Model file for the job. Use its own axes, mm. Coordinates: 2 decimals unless noted, no trailing zeros. Order: outer loops, then holes, each group sorted by start corner. A loop starts at its lowest first (then second) coordinate and runs counter-clockwise, first axis right, second up.
Autodesk Inventor part; units mm, degrees
ref_plane "YZ Plane" through (0, 0, 0) normal (1, 0, 0) x (0, 1, 0)
ref_plane "XZ Plane" through (0, 0, 0) normal (0, 1, 0) x (-1, 0, 0)
ref_plane "XY Plane" through (0, 0, 0) normal (0, 0, 1) x (1, 0, 0)
sketch "Sketch1" plane through (0, 0, 0) normal (0, 1, 0) x (-1, 0, 0)
  line L0 (0, 0) -> (63, 0)
  line L1 (63, 0) -> (63, -63)
  line L2 (63, -63) -> (0, -63)
  line L3 (0, -63) -> (0, 0)
  circle A0 centre (31.5, -31.5) radius 3.1
  circle A1 centre (12.45, -12.45) radius 2.5
  circle A2 centre (31.5, -12.45) radius 2.5
  circle A3 centre (50.55, -12.45) radius 2.5
  circle A4 centre (12.45, -50.55) radius 2.5
  circle A5 centre (31.5, -50.55) radius 2.5
  circle A6 centre (50.55, -50.55) radius 2.5
  point P0 (31.5, -63)
  dimension "d0" = 63
  dimension "d1" = 63
  dimension "d2" = 6.2
  dimension "d3" = 31.5
  dimension "d4" = 31.5
  dimension "d5" = 19.05
  dimension "d6" = 19.05
  dimension "d7" = 5
  dimension "d10" = 19.05
  dimension "d13" = 38.1
extrude "Extrusion1" add sketch "Sketch1" along normal blind 12 contours L0 L1 L2 L3 | A0
sketch "Sketch2" plane through (0, 12, 0) normal (0, 1, 0) x (1, 0, 0)
  circle A0 centre (-45, 31.5) radius 2.75
  circle A1 centre (-31.5, 31.5) radius 3.1
  circle A2 centre (-38.25, 19.8087) radius 2.75
  circle A3 centre (-24.75, 19.8087) radius 2.75
  circle A4 centre (-18, 31.5) radius 2.75
  circle A5 centre (-24.75, 43.1913) radius 2.75
  circle A6 centre (-38.25, 43.1913) radius 2.75
  point P0 (0, 0)
  dimension "d18" = 5.5
  dimension "d19" = 13.5
  dimension "d20" = 0
  dimension "d23" = 360
extrude "Extrusion2" cut sketch "Sketch2" against normal blind 12 contours A0 | A2 | A3 | A4 | A5 | A6
chamfer "Chamfer1" distance 3 angle 45 6 edges at (-41, 12, -43.1913) (-47.75, 12, -31.5) (-41, 12, -19.8087) (-27.5, 12, -19.8087) (-20.75, 12, -31.5) (-27.5, 12, -43.1913)
thread "Thread2"
thread "Thread3"
thread "Thread4"
thread "Thread5"
thread "Thread6"
thread "Thread7"
equation "\"d4\" = 0.5 * d0"
properties part number "Adapter plate for tube dovetail bracket"
Q1. Cut at A-A, the plane x = -45. List the corners of the cut face in (y, z), plus the area to 3 significant figures.
Established:
outline: (0, -63) - (12, -63) - (12, -37.25) - (9, -34.25) - (0, -34.25) - close; (0, -28.75) - (9, -28.75) - (12, -25.75) - (12, 0) - (0, 0) - close
area: 681 mm2
Q2. Mould opens along X. For faces 1 (the face through (-32, 6, -63)), 2 (the face through (-12.12, 5.92, -14.93)), 3 (the face through (-63, 6, -31)) say: pulls with the +X half, pulls with the -X half, needs draft (parallel to the pull), parting line crosses it, or undercut.
Established:
face 1: needs draft
face 2: undercut
face 3: pulls with the -X half
Q3. Probe line 1 (X direction, y = 1.25, z = -43); line 2 (Z direction, x = -38.25, y = 5.5); line 3 (Z direction, x = -31.5, y = 4). List the from-to ranges inside material, lowest first.
Established:
line 1: x = -63 to -40.99, -35.51 to -27.49, -22.01 to 0
line 2: z = -63 to -45.94, -40.44 to -22.56, -17.06 to 0
line 3: z = -63 to -53.05, -48.05 to -14.95, -9.95 to 0
Q4. Drop a flat-ended pin along its axis: P1, Ø4.5, axis at x = -18, z = -31.5, coming from the -Y side. Give the stop position or say it passes through.
Established:
P1: passes through
Q5. Cut at C-C, the plane z = -12.45. List the corners of the cut face in (x, y).
Established:
outline: (-63, 0) - (-53.05, 0) - (-53.05, 12) - (-63, 12) - close; (-48.05, 0) - (-34, 0) - (-34, 12) - (-48.05, 12) - close; (-29, 0) - (-14.95, 0) - (-14.95, 12) - (-29, 12) - close; (-9.95, 0) - (0, 0) - (0, 12) - (-9.95, 12) - close
Q6. Cut at D-D, the plane x = -24.75. List the corners of the cut face in (y, z), plus the area to 3 significant figures.
Established:
outline: (0, -63) - (12, -63) - (12, -48.94) - (9, -45.94) - (0, -45.94) - close; (0, -40.44) - (9, -40.44) - (12, -37.44) - (12, -25.56) - (9, -22.56) - (0, -22.56) - close; (0, -17.06) - (9, -17.06) - (12, -14.06) - (12, 0) - (0, 0) - close
area: 606 mm2
Q7. Cut at B-B, the plane z = -31.5. List the corners of the cut face in (x, y).
Established:
outline: (-63, 0) - (-47.75, 0) - (-47.75, 9) - (-50.75, 12) - (-63, 12) - close; (-42.25, 0) - (-20.75, 0) - (-20.75, 9) - (-23.75, 12) - (-39.25, 12) - (-42.25, 9) - close; (-15.25, 0) - (0, 0) - (0, 12) - (-12.25, 12) - (-15.25, 9) - close
